Check sheet for the modelled part. Datum: model origin and axes. Units: mm. A direction names the side the tool comes from. Give positions to 0.01 mm unless a question says otherwise; leave off trailing zeros. Order: outer loops, then holes, each group sorted by start corner. A loop starts at its lowest first (then second) coordinate and runs counter-clockwise, first axis right, second up. Notation, with made-up numbers: (-11.5, -14.75) - (47.5, -14.75) arc R22 ccw to (47.5, -0.75) - close; hole circle Ø11 at (-27.75, -22.5). An arc over 180 degrees is marked (long way). Answer in a Markdown table with one row per item.
from build123d import *

# Parameters (mm, degrees)
F0_W     = 90
F0_H     = 90
F1_DEPTH = 2.75
F3_DEPTH = 4
F4_R     = 2.25
F5_DEPTH = 5.501
F7_D     = 4.5


with BuildPart() as f1:
    # F0 (on Front) → F1 (new body, symmetric)
    with BuildSketch(Plane.XZ):
        Rectangle(F0_W, F0_H)
    extrude(amount=F1_DEPTH, both=True)

    # F2 (on face) → F3 (cut)
    with BuildSketch(Plane.XZ.offset(2.75)):
        Polygon((-16.334936, 9.75), (-20.665064, 9.75), (-22.830127, 6), (-20.665064, 2.25), (-16.334936, 2.25), (-14.169873, 6), align=None)
        Polygon((-16.334936, -2.25), (-20.665064, -2.25), (-22.830127, -6), (-20.665064, -9.75), (-16.334936, -9.75), (-14.169873, -6), align=None)
        Polygon((20.665064, -2.25), (16.334936, -2.25), (14.169873, -6), (16.334936, -9.75), (20.665064, -9.75), (22.830127, -6), align=None)
        Polygon((16.334936, 2.25), (20.665064, 2.25), (22.830127, 6), (20.665064, 9.75), (16.334936, 9.75), (14.169873, 6), align=None)
    extrude(amount=-F3_DEPTH, mode=Mode.SUBTRACT)

    # F4 (on face) → F5 (cut, through all)
    with BuildSketch(Plane.XZ.offset(2.75)):
        with Locations((-18.5, 6)):
            Circle(F4_R)
        with Locations((-18.5, -6)):
            Circle(F4_R)
        with Locations((18.5, 6)):
            Circle(F4_R)
        with Locations((18.5, -6)):
            Circle(F4_R)
    extrude(amount=-F5_DEPTH, mode=Mode.SUBTRACT)

    # F7 (through all)
    with Locations(Plane.XZ.offset(2.75)):
        with Locations((-40, 39), (-30, 39), (-20, 39), (-10, 39), (10, 39), (20, 39), (30, 39), (40, 39), (40, 29), (30, 29), (20, 29), (-10, 29), (10, 29), (-30, 29), (-20, 29), (-40, 29), (30, 19), (-40, 19), (10, 19), (-10, 19), (20, 19), (-20, 19), (40, 19), (-30, 19), (30, 10), (30, -10), (40, -39), (40, 10), (30, -29), (30, -39), (40, -19), (40, -10), (30, -19), (40, -29), (-30, -10), (-40, -19), (-40, -29), (-30, -19), (-30, -39), (-30, 10), (-40, -10), (-40, -39), (-40, 10), (-30, -29), (-10, -29), (20, -39), (-10, -19), (20, -29), (10, -19), (10, -29), (-20, -19), (-20, -39), (10, -39), (-10, -39), (-20, -29), (20, -19)):
            Hole(F7_D / 2)


solid = f1.part
(1) Thickness scan on L1, parallel to Y at x = 21, z = -3.5. Record the ranges inside material, lowest first.
Geometry says:
| item | result |
|---|---|
| L1 | 1.25 to 2.75 |
(2) Cross-section at A-A, the plane x = 10. Record the cut outline in (y, z).
Geometry says:
| item | result |
|---|---|
| outline | (-2.75, -45) - (2.75, -45) - (2.75, -41.25) - (-2.75, -41.25) - close; (-2.75, -36.75) - (2.75, -36.75) - (2.75, -31.25) - (-2.75, -31.25) - close; (-2.75, -26.75) - (2.75, -26.75) - (2.75, -21.25) - (-2.75, -21.25) - close; (-2.75, -16.75) - (2.75, -16.75) - (2.75, 16.75) - (-2.75, 16.75) - close; (-2.75, 21.25) - (2.75, 21.25) - (2.75, 26.75) - (-2.75, 26.75) - close; (-2.75, 31.25) - (2.75, 31.25) - (2.75, 36.75) - (-2.75, 36.75) - close; (-2.75, 41.25) - (2.75, 41.25) - (2.75, 45) - (-2.75, 45) - close |
(3) Cross-section at B-B, the plane z = 39. Give the number of separate pieces and of enclosed holes in the cut face, then the cut area to 3 significant figures.
Geometry says:
| item | result |
|---|---|
| separate pieces | 9 |
| enclosed holes | 0 |
| area | 297 mm² |
(4) Gauge pin test, flat ends, axial feed: P1, Ø2.5, axis at x = -20, z = 29, coming from the -Y side; P2, Ø2, axis at x = 17.5, z = -5, coming from the -Y side. Record the tip position at first contact, or that the pin passes through.
Geometry says:
| item | result |
|---|---|
| P1 | through |
| P2 | y = 1.25 |
(5) Access from +Z, -Z, +X, -X, +Y, -Y to the whole of each face (thin tool, end or side, straight path). Record for faces 1 (the flat face through (19, -1, 9.75)), 2 (the cylindrical face through (-21.038, 0.038, -20.996)).
Geometry says:
| item | result |
|---|---|
| face 1 | -Y |
| face 2 | +Y, -Y |
